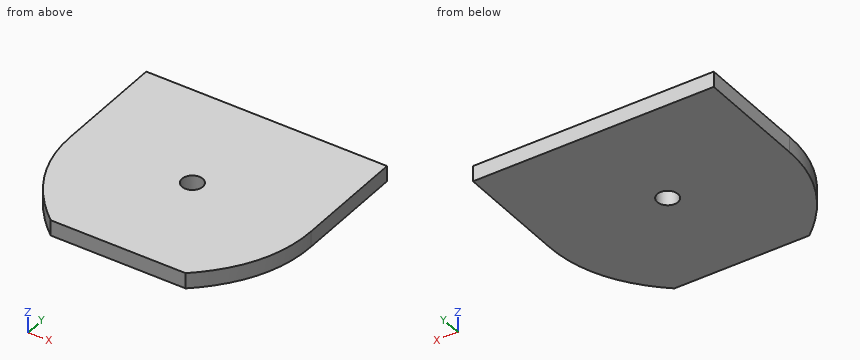
```python
from build123d import *

# Parameters (mm, degrees)
BOSS_EXTRUDE1_DEPTH = 0.75
CUT_EXTRUDE1_REACH  = 14.106
SKETCH2_R           = 0.5


with BuildPart() as part:
    # Sketch1 → Boss-Extrude1 (new body)
    with BuildSketch(Plane.XY):
        with BuildLine():
            Line((-3.25, 0), (3.25, 0))
            add(Edge.make_bspline(
                [(5.8, 5.176744099), (5.8, 3.033630296), (4.795112478, 1.311398784), (3.25, 0)],
                knots=[0, 0, 0, 0, 1, 1, 1, 1], degree=3))
            Line((5.8, 5.176744099), (5.8, 10.6))
            Line((5.8, 10.6), (-5.8, 10.6))
            Line((-5.8, 10.6), (-5.8, 5.176744099))
            add(Edge.make_bspline(
                [(-5.8, 5.176744099), (-5.8, 3.033630296), (-4.795112478, 1.311398784), (-3.25, 0)],
                knots=[0, 0, 0, 0, 1, 1, 1, 1], degree=3))
        make_face()
    extrude(amount=BOSS_EXTRUDE1_DEPTH)

    # Sketch2 → Cut-Extrude1 (cut, up to next)
    with BuildSketch(Plane.XY.offset(0.75), mode=Mode.PRIVATE) as cut_extrude1_sk1:
        with Locations((0, 5.3)):
            Circle(SKETCH2_R)
    cut_extrude1_tool1 = extrude(cut_extrude1_sk1.sketch, amount=-CUT_EXTRUDE1_REACH, mode=Mode.PRIVATE) & part.part
    add(cut_extrude1_tool1.solids().sort_by_distance((0, 5.3, 0.75))[0], mode=Mode.SUBTRACT)


solid = part.part
```
Here's how the part is built. I have some questions about the finished solid (model axes, mm). Round coordinates to 2 decimals unless told otherwise and drop trailing zeros. Order: outer loops, then holes, each group sorted by start corner. A loop starts at its lowest first (then second) coordinate and runs counter-clockwise, first axis right, second up. Notation, with made-up numbers: (25, 7) -> (45, 7) arc R22 cw to (45, 46) -> close; hole circle Ø3 at (24.5, 26). An arc over 180 degrees is marked (long way). Use a Markdown table: item, result. Add a question column.
(1) I need wall thicknesses on line 1 along Y through (x, z) = (0, 0.35); line 2 along X through (y, z) = (5, 0.55); line 3 along X through (y, z) = (3.75, 0.2). Which ranges of each line are inside material? Lowest first, please.
(2) Suppose I cut it at A-A, the plane x = 0. Please give me the cut outline in (y, z).
(3) For pin 1 Ø3 at (x, y) = (3.5, 4) entering from -Z, with a flat end and sliding along its axis, tell me the tip position at first contact or that it passes through.
Verdict:
| question | item | result |
|---|---|---|
| 1 | line 1 | 0 to 4.8, 5.8 to 10.6 |
| 1 | line 2 | -5.8 to -0.4, 0.4 to 5.8 |
| 1 | line 3 | -5.64 to 5.64 |
| 2 | outline | (0, 0) -> (4.8, 0) -> (4.8, 0.75) -> (0, 0.75) -> close; (5.8, 0) -> (10.6, 0) -> (10.6, 0.75) -> (5.8, 0.75) -> close |
| 3 | pin 1 | z = 0 |
